from build123d import *

# Parameters (mm, degrees)
SKETCH_1_R      = 1.4
SKETCH_1_W      = 21
SKETCH_1_H      = 42
EXTRUDE_1_DEPTH = 6
FILLET_6_R      = 3
FILLET_7_R      = 3
FILLET_8_R      = 3
FILLET_9_R      = 3
FILLET_10_R     = 3
FILLET_11_R     = 3
SKETCH_2_R      = 2.5
EXTRUDE_2_DEPTH = 2


with BuildPart() as part:
    # 草圖1 → 填料-伸長1 (new body)
    with BuildSketch(Plane.XY):
        with BuildLine():
            Line((8, -18.141285654), (8, 17.94275172))
            ThreePointArc((8, 17.94275172), (0, 21.985231559), (-8, 17.94275172))
            Line((-8, 17.94275172), (-8, -18.141285654))
            Line((-8, -18.141285654), (-8, -28.206652459))
            Line((-8, -28.206652459), (-12.5, -28.206652459))
            Line((-12.5, -28.206652459), (-12.5, -81.793347541))
            Line((-12.5, -81.793347541), (12.5, -81.793347541))
            Line((12.5, -81.793347541), (12.5, -28.206652459))
            Line((12.5, -28.206652459), (8, -28.206652459))
            Line((8, -28.206652459), (8, -18.141285654))
        make_face()
        with Locations((-4.7, -78.8)):
            Circle(SKETCH_1_R, mode=Mode.SUBTRACT)
        with Locations((0, -55)):
            Rectangle(SKETCH_1_W, SKETCH_1_H, mode=Mode.SUBTRACT)
        with Locations((-4.7, -31.2)):
            Circle(SKETCH_1_R, mode=Mode.SUBTRACT)
        with Locations((4.7, -78.8)):
            Circle(SKETCH_1_R, mode=Mode.SUBTRACT)
        with Locations((4.7, -31.2)):
            Circle(SKETCH_1_R, mode=Mode.SUBTRACT)
        with BuildLine():
            ThreePointArc((-4.999271035, -4.154189345), (-6.5, 0), (-4.999271035, 4.154189345))
            Line((-4.999271035, 4.154189345), (-2.6, 17.94275172))
            ThreePointArc((-2.6, 17.94275172), (0, 20), (2.6, 17.94275172))
            Line((2.6, 17.94275172), (4.999271035, 4.154189345))
            ThreePointArc((4.999271035, 4.154189345), (6.5, 0), (4.999271035, -4.154189345))
            Line((4.999271035, -4.154189345), (2.6, -17.94275172))
            ThreePointArc((2.6, -17.94275172), (0, -20), (-2.6, -17.94275172))
            Line((-2.6, -17.94275172), (-4.999271035, -4.154189345))
        make_face(mode=Mode.SUBTRACT)
    extrude(amount=EXTRUDE_1_DEPTH)

    # 圓角6
    fillet_6_edges = [part.edges().sort_by_distance(p)[0] for p in [
        (-12.5, -81.793347541, 3),
    ]]
    fillet(fillet_6_edges, radius=FILLET_6_R)

    # 圓角7
    fillet_7_edges = [part.edges().sort_by_distance(p)[0] for p in [
        (12.5, -81.793347541, 3),
    ]]
    fillet(fillet_7_edges, radius=FILLET_7_R)

    # 圓角8
    fillet_8_edges = [part.edges().sort_by_distance(p)[0] for p in [
        (12.5, -28.206652459, 3),
    ]]
    fillet(fillet_8_edges, radius=FILLET_8_R)

    # 圓角9
    fillet_9_edges = [part.edges().sort_by_distance(p)[0] for p in [
        (8, -28.206652459, 3),
    ]]
    fillet(fillet_9_edges, radius=FILLET_9_R)

    # 圓角10
    fillet_10_edges = [part.edges().sort_by_distance(p)[0] for p in [
        (-12.5, -28.206652459, 3),
    ]]
    fillet(fillet_10_edges, radius=FILLET_10_R)

    # 圓角11
    fillet_11_edges = [part.edges().sort_by_distance(p)[0] for p in [
        (-8, -28.206652459, 3),
    ]]
    fillet(fillet_11_edges, radius=FILLET_11_R)

    # 草圖2 → 填料-伸長2 (add)
    with BuildSketch(Plane.XY):
        with BuildLine():
            Line((-3.702325647, 20.172267208), (4.497563026, 20.172267208))
            ThreePointArc((4.497563026, 20.172267208), (6.068658829, 19.068237677), (7.032818959, 17.407629814))
            Line((7.032818959, 17.407629814), (7.032818959, -20.628324178))
            Line((7.032818959, -20.628324178), (-6.646673958, -20.628324178))
            Line((-6.646673958, -20.628324178), (-6.646673958, 17.471058727))
            ThreePointArc((-6.646673958, 17.471058727), (-5.621736824, 19.309156464), (-3.702325647, 20.172267208))
        make_face()
        Circle(SKETCH_2_R, mode=Mode.SUBTRACT)
    extrude(amount=EXTRUDE_2_DEPTH)


solid = part.part
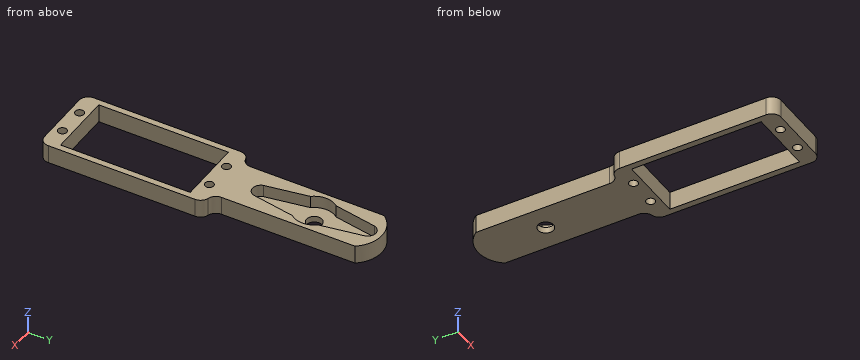
Verification items for the finished model (mm, model axes). Round coordinates to 2 decimals unless told otherwise and drop trailing zeros. Write each loop counter-clockwise with the first axis right and the second up, starting at its lowest first coordinate (ties: lowest second). Pieces come first, ordered by that corner, then holes.
(1) Section check C-C (y = -8.5). Enter the section's corners in (x, z).
Returned:
outline: (-8, 0) - (8, 0) - (8, 6) - (4.24, 6) - (4.24, 2) - (-4.24, 2) - (-4.24, 6) - (-8, 6) - close
(2) Section check D-D (z = 5). Give the number of separate pieces and of enclosed holes in the cut face, plus the area to 3 significant figures.
Returned:
separate pieces: 1
enclosed holes: 6
area: 886 mm2
(3) Section check A-A (y = -36). Enter the section's corners in (x, z).
Returned:
outline: (-12.5, 0) - (-10.5, 0) - (-10.5, 6) - (-12.5, 6) - close; (10.5, 0) - (12.5, 0) - (12.5, 6) - (10.5, 6) - close
(4) Depth check by flat-ended pin: pin 1 Ø3.5 at (x, y) = (4.7, -31.2) entering from +Z; pin 2 Ø6.5 at (x, y) = (1, 4.5) entering from +Z; pin 3 Ø3 at (y, z) = (1, 3.5) entering from -X; pin 4 Ø3 at (y, z) = (5, 1.5) entering from +X. Enter the tip coordinate at first touch or a pass-through.
Returned:
pin 1: stops at z = 6
pin 2: stops at z = 2
pin 3: stops at x = -8
pin 4: stops at x = 8
(5) Material ranges on line 1 (Y direction, x = 0, z = 1.4); line 2 (X direction, y = -32, z = 2.5); line 3 (Y direction, x = 2, z = 5.75), recorded low to high.
Returned:
line 1: y = -81.79 to -76, -34 to -2.5, 2.5 to 21.99
line 2: x = -12.5 to -5.85, -3.55 to 3.55, 5.85 to 12.5
line 3: y = -81.79 to -76, -34 to -19.1, 19.1 to 21.78
(6) Section check B-B (x = 0). Enter the section's corners in (y, z).
Returned:
outline: (-81.79, 0) - (-76, 0) - (-76, 6) - (-81.79, 6) - close; (-34, 0) - (-2.5, 0) - (-2.5, 2) - (-20, 2) - (-20, 6) - (-34, 6) - close; (2.5, 0) - (21.99, 0) - (21.99, 6) - (20, 6) - (20, 2) - (2.5, 2) - close
